Read the model definition and answer for the solid it produces. Units are mm, in the model's axes. Face numbers are marked on the shaded views. A direction names the side the tool comes from. Round coordinates to 2 decimals unless told otherwise and drop trailing zeros. Order: outer loops, then holes, each group sorted by start corner. A loop starts at its lowest first (then second) coordinate and runs counter-clockwise, first axis right, second up.
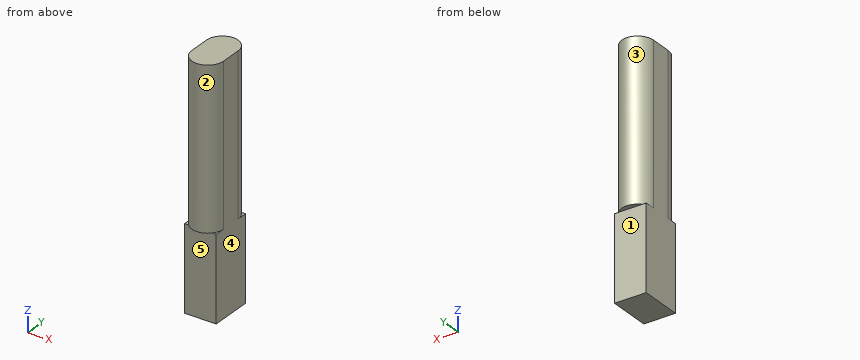
Autodesk Inventor part; units mm, degrees
ref_plane "YZ Plane" through (0, 0, 0) normal (1, 0, 0) x (0, 1, 0)
ref_plane "XZ Plane" through (0, 0, 0) normal (0, 1, 0) x (-1, 0, 0)
ref_plane "XY Plane" through (0, 0, 0) normal (0, 0, 1) x (1, 0, 0)
sketch "Sketch1" plane through (0, 0, 0) normal (0, 0, 1) x (1, 0, 0)
  line L0 (0, 0) -> (3, 0)
  line L1 (3, 0) -> (3, 4)
  line L2 (3, 4) -> (0, 4)
  line L3 (0, 4) -> (0, 0)
  dimension "d0" = 3
  dimension "d1" = 4
extrude "Extrusion1" add sketch "Sketch1" along normal blind 4
sketch "Sketch2" plane through (0, 0, 4) normal (0, 0, 1) x (1, 0, 0)
  line L0 (0, 0) -> (3, 0)
  line L1 (3, 0) -> (3, 4)
  line L2 (3, 4) -> (0, 4)
  line L3 (0, 4) -> (0, 0)
  dimension "d4" = 3
  dimension "d5" = 4
extrude "Extrusion2" add sketch "Sketch2" along normal blind 4
sketch "Sketch3" plane through (0, 0, 8) normal (0, 0, 1) x (1, 0, 0)
  line L0 (1.5, -0.5) -> (1.5, -0.5)
  line L1 (3, 1) -> (3, 3)
  line L2 (1.5, 4.5) -> (1.5, 4.5)
  line L3 (0, 3) -> (0, 1)
  arc A0 (1.5, 4.5) -> (0, 3) centre (1.5, 3) ccw
  arc A1 (0, 1) -> (1.5, -0.5) centre (1.5, 1) ccw
  arc A2 (1.5, -0.5) -> (3, 1) centre (1.5, 1) ccw
  arc A3 (3, 3) -> (1.5, 4.5) centre (1.5, 3) ccw
  point P0 (0, 0)
  point P1 (3, 4.5)
  point P2 (3, -0.5)
  point P3 (0, 4.5)
  dimension "d8" = 3
  dimension "d9" = 5
  dimension "d10" = 1.5
  dimension "d11" = 1.5
extrude "Extrusion3" add sketch "Sketch3" along normal blind 15
properties part number "button_press"
Q1. A cutting plane is placed at B-B, the plane z = 16.75. Give the vertices of the cut face in (x, y).
Outcome:
outline: (0, 1) arc R1.5 ccw to (3, 1) - (3, 3) arc R1.5 ccw to (0, 3) - close
Q2. A cutting plane is placed at D-D, the plane z = 5. Give the vertices of the cut face in (x, y), plus the area to 3 significant figures.
Outcome:
outline: (0, 0) - (3, 0) - (3, 4) - (0, 4) - close
area: 12.0 mm2
Q3. A cutting plane is placed at A-A, the plane x = 0.9. Give the vertices of the cut face in (y, z).
Outcome:
outline: (-0.37, 8) - (0, 8) - (0, 0) - (4, 0) - (4, 8) - (4.37, 8) - (4.37, 23) - (-0.37, 23) - close
Q4. Straight lines are drawn through the part: probe 1 along Y at (x, z) = (0.5, 5.75); probe 2 along Y at (x, z) = (1.4, 16.75); probe 3 along Z at (x, y) = (1.35, 4.35). For each, find the intervals that lie inside material, in ascending order.
Outcome:
probe 1: y = 0 to 4
probe 2: y = -0.5 to 4.5
probe 3: z = 8 to 23
Q5. For the marked faces 1, 2, 3, 4 and 5, determine the directions among +Z, -Z, +X, -X, +Y, -Y from which every point of the face is accessible in a straight line to the end or side of a thin tool.
Outcome:
face 1: -Z, +X, -X, +Y
face 2: +Z, -Y
face 3: +Z, +Y
face 4: +Z, -Z, +X, +Y, -Y
face 5: -Z, +X, -X, -Y
Q6. A cutting plane is placed at C-C, the plane x = 2.3. Give the vertices of the cut face in (y, z), plus the area to 3 significant figures.
Outcome:
outline: (-0.27, 8) - (0, 8) - (0, 0) - (4, 0) - (4, 8) - (4.27, 8) - (4.27, 23) - (-0.27, 23) - close
area: 100 mm2
Q7. Flat-ended cylindrical pins translate along their axes: pin 1 (0.9 mm diameter, centred on x = 1, z = 4.5, fed in from +Y); pin 2 (1.5 mm diameter, centred on x = 2, z = 3, fed in from -Y). Find the tip coordinate at first contact, or state that the pin passes through.
Outcome:
pin 1: stops at y = 4
pin 2: stops at y = 0
